```python
from build123d import *

# Parameters (mm, degrees)
SKETCH2_W           = 12.7
SKETCH2_H           = 15.875
BOSS_EXTRUDE1_DEPTH = 3.81
SKETCH3_R           = 1.397
CUT_EXTRUDE1_DEPTH  = 3.81
SKETCH6_R           = 2.694076836
BOSS_EXTRUDE2_DEPTH = 3.81
SKETCH8_R           = 1.27
CUT_EXTRUDE3_DEPTH  = 1.778
BOSS_EXTRUDE3_START = -3.81
SKETCH9_R           = 2.694076836
BOSS_EXTRUDE3_DEPTH = 3.81
CUT_EXTRUDE4_START  = -1.778
SKETCH10_R          = 1.27
CUT_EXTRUDE4_DEPTH  = 1.778


with BuildPart() as part:
    # Sketch2 → Boss-Extrude1 (new body)
    with BuildSketch(Plane(origin=(0, 0, 0), x_dir=(1, 0, 0), z_dir=(0, 1, 0))):
        with Locations((6.35, 7.9375)):
            Rectangle(SKETCH2_W, SKETCH2_H)
    extrude(amount=BOSS_EXTRUDE1_DEPTH)

    # Sketch3 → Cut-Extrude1 (cut)
    with BuildSketch(Plane(origin=(0, 3.81, 0), x_dir=(1, 0, 0), z_dir=(0, 1, 0))):
        with Locations(Location((9.652, 3.81, 0), (0, 0, 270))):
            Circle(SKETCH3_R)
        with Locations(Location((9.652, 12.065, 0), (0, 0, 270))):
            Circle(SKETCH3_R)
    extrude(amount=-CUT_EXTRUDE1_DEPTH, mode=Mode.SUBTRACT)

    # Sketch6 → Boss-Extrude2 (add)
    with BuildSketch(Plane.XY):
        with Locations((-1.905, 1.905)):
            Circle(SKETCH6_R)
    extrude(amount=-BOSS_EXTRUDE2_DEPTH)

    # Sketch8 → Cut-Extrude3 (cut)
    with BuildSketch(Plane(origin=(0, 0, -3.81), x_dir=(-1, 0, 0), z_dir=(0, 0, -1))):
        with Locations((1.905, 1.905)):
            Circle(SKETCH8_R)
    extrude(amount=-CUT_EXTRUDE3_DEPTH, mode=Mode.SUBTRACT)

    # Sketch9 → Boss-Extrude3 (add)
    with BuildSketch(Plane(origin=(0, 0, -15.875), x_dir=(-1, 0, 0), z_dir=(0, 0, -1)).offset(BOSS_EXTRUDE3_START)):
        with Locations((1.905, 1.905)):
            Circle(SKETCH9_R)
    extrude(amount=BOSS_EXTRUDE3_DEPTH)

    # Sketch10 → Cut-Extrude4 (cut)
    with BuildSketch(Plane.XY.offset(-12.065).offset(CUT_EXTRUDE4_START)):
        with Locations(Location((-1.905, 1.905, 0), (0, 0, 180))):
            Circle(SKETCH10_R)
    extrude(amount=CUT_EXTRUDE4_DEPTH, mode=Mode.SUBTRACT)


solid = part.part
```
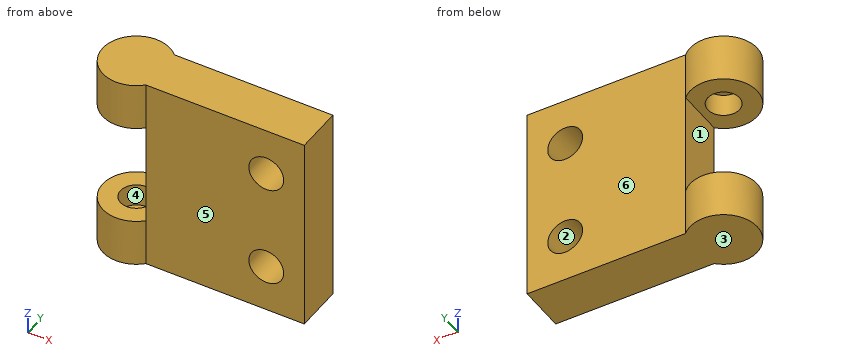
Part model, mm, in its own coordinate system. Face numbers are marked on the shaded views. A direction names the side the tool comes from. Round coordinates to 2 decimals unless told otherwise and drop trailing zeros. Write each loop counter-clockwise with the first axis right and the second up, starting at its lowest first coordinate (ties: lowest second). Pieces come first, ordered by that corner, then holes. Notation, with made-up numbers: M 31,71.5 L 81,71.5 A16 ccw 81,84.5 Z; hole C 19,58 d8. An arc over 180 degrees is marked long. One line per question, with ' | ' between items.
(1) Saw through at C-C on y = 4.35. Write the cut outline in (x, z) (3 decimals).
Answer key:
outline: M -3.036,-15.875 L -0.774,-15.875 L -0.774,-12.065 L -3.036,-12.065 Z; M -3.036,-3.81 L -0.774,-3.81 L -0.774,0 L -3.036,0 Z
(2) Probe line 1 along Z through (x, y) = (-0.75, 2.1) (3 decimals); line 2 along X through (y, z) = (3, -5.5); line 3 along Y through (x, z) = (10.75, -4.75). List the from-to ranges inside material, lowest first.
Answer key:
line 1: z = -15.875 to -13.843, -2.032 to 0 | line 2: x = 0 to 12.7 | line 3: y = 0 to 3.81
(3) Saw through at D-D on z = -1.25. Write the cut outline in (x, y) (3 decimals), then the cut area to 3 significant figures.
Answer key:
outline: M 0,0 L 12.7,0 L 12.7,3.81 L 0,3.81 A2.694 ccw long Z | area: 69.1 mm^2
(4) Saw through at A-A on y = 2.9. Write the cut outline in (x, z) (3 decimals), then the cut area to 3 significant figures.
Answer key:
outline: M -4.409,-15.875 L 12.7,-15.875 L 12.7,0 L -4.409,0 L -4.409,-3.81 L -2.694,-3.81 L -2.694,-2.032 L -1.116,-2.032 L -1.116,-3.81 L 0,-3.81 L 0,-12.065 L -1.116,-12.065 L -1.116,-13.843 L -2.694,-13.843 L -2.694,-12.065 L -4.409,-12.065 Z; hole C 9.652,-12.065 d2.794; hole C 9.652,-3.81 d2.794 | area: 217 mm^2
(5) Saw through at B-B on x = -2.75. Write the cut outline in (y, z) (3 decimals), then the cut area to 3 significant figures.
Answer key:
outline: M -0.653,-15.875 L 4.463,-15.875 L 4.463,-12.065 L 2.853,-12.065 L 2.853,-13.843 L 0.957,-13.843 L 0.957,-12.065 L -0.653,-12.065 Z; M -0.653,-3.81 L 0.957,-3.81 L 0.957,-2.032 L 2.853,-2.032 L 2.853,-3.81 L 4.463,-3.81 L 4.463,0 L -0.653,0 Z | area: 32.2 mm^2
(6) Pin check, flat tips, straight feed: pin 1 (6 mm diameter, centred on x = 5, z = -8, fed in from +Y); pin 2 (2 mm diameter, centred on x = 9.5, z = -7, fed in from -Y); pin 3 (1.7 mm diameter, centred on x = 9.652, z = -12.065, fed in from -Y). Stop position of each tip, or through.
Answer key:
pin 1: stops at y = 3.81 | pin 2: stops at y = 0 | pin 3: passes through
(7) 3-axis set-ups, long thin cutter, end or side, ignore diameter. For the marked faces 4, 5 and 6: which of +Z, -Z, +X, -X, +Y, -Y reach the whole face in a straight line?
Answer key:
face 4: none | face 5: +Z, -Z, +X, -Y | face 6: +Z, -Z, +X, +Y
(8) Two-plate mould, pull along X, no slides. Class the marked faces 1, 2 and 3: released by +X, released by -X, zero draft, split by the parting line, or undercut.
Answer key:
face 1: released by -X | face 2: undercut | face 3: zero draft
